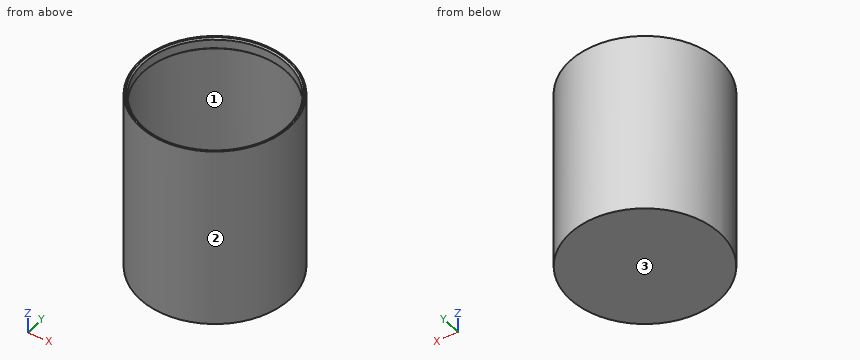
Autodesk Fusion 360 part; units mm, degrees
sketch "Sketch1" plane through (0, 0, 0) normal (0, 0, 1) x (1, 0, 0)
  circle A0 centre (0, 0) radius 50
extrude "Extrude1" add sketch "Sketch1" along normal blind 2
sketch "Sketch2" plane through (0, 0, 2) normal (0, 0, 1) x (-1, 0, 0)
  circle A0 centre (0, 0) radius 50
  circle A1 centre (0, 0) radius 49.5
  circle A2 centre (0, 0) radius 50
  dimension "d5" = 99
extrude "Extrude2" add sketch "Sketch2" along normal blind 120
sketch "Sketch3" plane through (0, 0, 122) normal (0, 0, 1) x (-1, 0, 0)
  circle A0 centre (0, 0) radius 49.5
  circle A1 centre (0, 0) radius 50
  circle A2 centre (0, 0) radius 48
  circle A3 centre (0, 0) radius 49.5
extrude "Extrude3" add sketch "Sketch3" against normal blind 8 contours A0 A3
chamfer "Chamfer1" distance 1 angle 45 2 edges at (44.7517, -17.3575, 122) (44.7517, 17.3575, 114)
Could you check a few things on this model? Use its own coordinates, in mm. Face numbers are marked on the shaded views. Coordinates: 2 decimals unless noted, no trailing zeros. Order: outer loops, then holes, each group sorted by start corner. A loop starts at its lowest first (then second) coordinate and runs counter-clockwise, first axis right, second up. Notation, with made-up numbers: (20.5, 61) -> (76.5, 61) arc R32 ccw to (76.5, 96) -> close; hole circle Ø4 at (56.25, -8.5). An arc over 180 degrees is marked (long way). One line per item, written item: value. Start each with the question number.
1) We'd pull the mould along X, two halves only. Please class the marked faces 1, 2 and 3: +X half, -X half, draft (parallel to the pull), parting line (faces both ways), or undercut.
2) If I drill on L1, parallel to Y at x = 0, z = 117.9; L2, parallel to X at y = 0, z = 74.5, over which ranges is the centre line in solid material (lowest first)? Write a range as [from, to].
3) I'm going to push flat-ended pins straight in: pin 1 (1 mm diameter, centred on y = 12.5, z = 66.5, fed in from -X); pin 2 (1 mm diameter, centred on y = 27.5, z = 25, fed in from -X); pin 3 (6 mm diameter, centred on x = 11, z = 66, fed in from +Y). Where does each tip first touch, or does it pass through?
4) Imagine slicing it at A-A on z = 64. List the corners of the cut face in (x, y) for me.
Answer list:
1. face 1: undercut
1. face 2: parting line
1. face 3: draft
2. L1: y = [-50, -48], [48, 50]
2. L2: x = [-50, -49.5], [49.5, 50]
3. pin 1: stops at x = -48.54
3. pin 2: stops at x = -42.08
3. pin 3: stops at y = 49.36
4. outline: circle Ø100 at (0, 0); hole circle Ø99 at (0, 0)
